Design review of the part built by this model. Coordinates are the model's own, in mm. Face numbers are marked on the shaded views. A direction names the side the tool comes from. Round coordinates to 2 decimals unless told otherwise and drop trailing zeros. Write each loop counter-clockwise with the first axis right and the second up, starting at its lowest first coordinate (ties: lowest second). Pieces come first, ordered by that corner, then holes. Notation, with made-up numbers: (87, 35) - (132, 35) arc R30 cw to (132, 59) - close; hole circle Ø9 at (42.5, 74). An arc over 180 degrees is marked (long way). Use one line per item in the form item = value.
```python
from build123d import *

# Parameters (mm, degrees)
F0_R     = 6.35
F1_DEPTH = 16.002
F2_DEPTH = 38.1
F4_DEPTH = 25.4


with BuildPart() as f1:
    # F0 (on Front) → F1 (new body)
    with BuildSketch(Plane.XZ):
        with BuildLine():
            Line((-109.882609, 44.45), (-109.882609, 15.558309))
            Line((-109.882609, 15.558309), (-59.544396, 15.558309))
            ThreePointArc((-59.544396, 15.558309), (-78.025435, 24.116231), (-84.524632, 43.417714))
            ThreePointArc((-84.524632, 43.417714), (-96.666039, 57.13949), (-109.882609, 44.45))
        make_face()
        with Locations((-97.182609, 44.45)):
            Circle(F0_R, mode=Mode.SUBTRACT)
        with BuildLine():
            Line((-59.544396, 15.558309), (-8.287901, 15.558309))
            Line((-8.287901, 15.558309), (-8.287901, 44.816575))
            ThreePointArc((-8.287901, 44.816575), (-20.982609, 57.15), (-33.677318, 44.816575))
            ThreePointArc((-33.677318, 44.816575), (-41.311473, 25.502285), (-59.544396, 15.558309))
        make_face()
        with Locations((-20.982609, 44.45)):
            Circle(F0_R, mode=Mode.SUBTRACT)
    extrude(amount=F1_DEPTH)

    # F0 (on Front) → F2 (join)
    with BuildSketch(Plane.XZ):
        Polygon((-109.882609, 15.558309), (-109.882609, 0), (-8.287901, 0), (-8.287901, 15.558309), (-59.544396, 15.558309), align=None)
    extrude(amount=F2_DEPTH)

    # F3 (on face) → F4 (cut)
    with BuildSketch(Plane.XY.offset(15.558309)):
        with BuildLine():
            Line((-40.037901, -21.03122), (-78.137901, -21.03122))
            ThreePointArc((-78.137901, -21.03122), (-84.487901, -27.38122), (-78.137901, -33.73122))
            Line((-78.137901, -33.73122), (-40.037901, -33.73122))
            ThreePointArc((-40.037901, -33.73122), (-33.687901, -27.38122), (-40.037901, -21.03122))
        make_face()
    extrude(amount=-F4_DEPTH, mode=Mode.SUBTRACT)


solid = f1.part
```
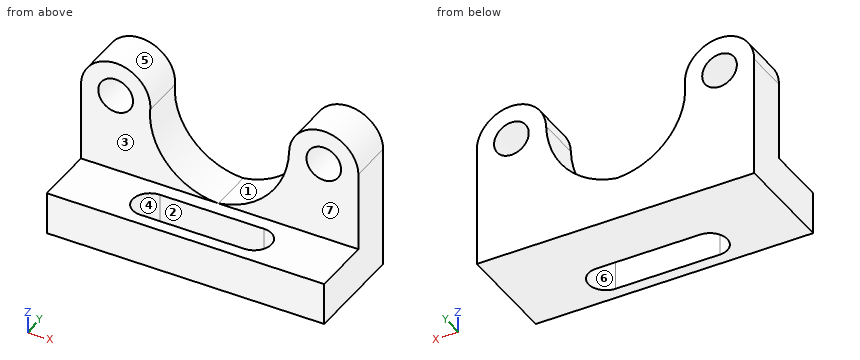
Q1. Machinability: for the marked faces 1, 2 and 3, which of the approach directions +Z, -Z, +X, -X, +Y, -Y give a long, thin tool a straight path to every point of the face, cutting with its end or side? Answer none if there is none.
Calculated:
face_1 = +Z, +Y, -Y
face_2 = +Z, -Z
face_3 = +Z, +X, -X, -Y
Q2. We need section D-D on z = 14. Write out the cut boundary in (x, y).
Calculated:
outline = (-109.88, -38.1) - (-8.29, -38.1) - (-8.29, 0) - (-109.88, 0) - close; hole (-78.14, -33.73) - (-40.04, -33.73) arc R6.35 ccw to (-40.04, -21.03) - (-78.14, -21.03) arc R6.35 ccw to start
Q3. We need section A-A on z = 22. Write out the cut boundary in (x, y).
Calculated:
outline = (-109.88, -16) - (-75.89, -16) - (-75.89, 0) - (-109.88, 0) - close; (-44.97, -16) - (-8.29, -16) - (-8.29, 0) - (-44.97, 0) - close
Q4. To check wall thickness, follow line 1 along X through (y, z) = (-10, 44); line 2 along Y through (x, z) = (-76.5, 7); line 3 along Y through (x, z) = (-97.5, 27). State the ranges of each line that lie inside material, in increasing order. Write a range as from..to.
Calculated:
line_1 = -109.88..-103.52, -90.85..-84.49, -33.71..-27.32, -14.65..-8.29
line_2 = -38.1..-33.73, -21.03..0
line_3 = -16..0
Q5. We need section C-C on x = -20.5. Write out the cut boundary in (y, z).
Calculated:
outline = (-38.1, 0) - (0, 0) - (0, 38.12) - (-16, 38.12) - (-16, 15.56) - (-38.1, 15.56) - close; (-16, 50.78) - (0, 50.78) - (0, 57.14) - (-16, 57.14) - close
Q6. We need section B-B on y = -30. Write out the cut boundary in (x, z), then the cut area to 3 significant figures.
Calculated:
outline = (-109.88, 0) - (-83.92, 0) - (-83.92, 15.56) - (-109.88, 15.56) - close; (-34.25, 0) - (-8.29, 0) - (-8.29, 15.56) - (-34.25, 15.56) - close
area = 808 mm2
Q7. Draft analysis for pull direction Y (two halves, no side actions). For the marked faces 4, 5, 6 and 7, state which applies: released by +Y, released by -Y, zero draft, split by the parting line, or undercut.
Calculated:
face_4 = undercut
face_5 = zero draft
face_6 = undercut
face_7 = released by -Y
Q8. For P1, Ø21, axis at x = -76, z = 27.5, coming from the -Y side; P2, Ø10, axis at x = -59, y = -12, coming from the +Z side; P3, Ø12, axis at x = -56, y = -4.5, coming from the +Z side, all flat-tipped, find the tip position at first contact; note any pin that passes through.
Calculated:
P1 = -16
P2 = 16.95
P3 = 18.69
